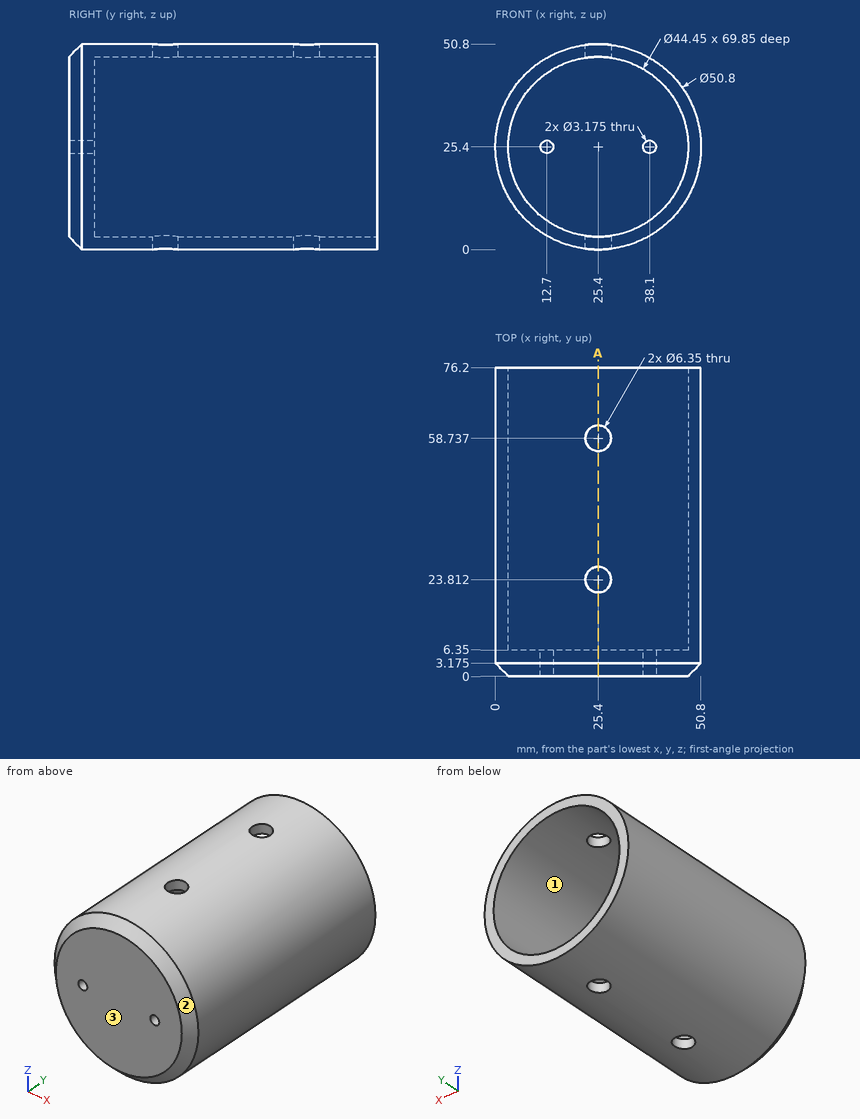
Study the drawing (mm; zero at the part's minimum x, y, z) and answer. Round coordinates to 2 decimals unless told otherwise and drop trailing zeros. Return JSON: item names as keys, results as strings. Group by question number.
Q1. Find the intervals of material crossed by L1, parallel to Y at x = 25.4, z = 2.65 (1 decimal); L2, parallel to Y at x = 12, z = 37; L3, parallel to X at y = 13, z = 5.5 (1 decimal), in increasing order.
Q2. The part is cut by section A-A on x = 25.4. Count the separate pieces of the cut face and the enclosed holes in it.
Q3. The mould has two halves that part along X. Classify the marked faces 1, 2 and 3: released by +X, released by -X, zero draft, split by the parting line, or undercut.
Q4. Each of these flat-tipped pins is pushed along its axis until it touches: pin 1 Ø12 at (x, y) = (36.5, 36.5) entering from +Z; pin 2 Ø22 at (x, z) = (26.5, 24.5) entering from +Y; pin 3 Ø6 at (y, z) = (43, 41.5) entering from -X. Where does it stop, or does it pass through?
Solved:
{
 "1": {"L1": "0.5 to 20.6, 27 to 55.6, 61.9 to 76.2", "L2": "0 to 6.35", "L3": "9.6 to 15.5, 35.3 to 41.2"},
 "2": {"separate pieces": "5", "enclosed holes": "0"},
 "3": {"face 1": "undercut", "face 2": "split by the parting line", "face 3": "zero draft"},
 "4": {"pin 1": "z = 50.28", "pin 2": "y = 6.35", "pin 3": "x = 3.64"}
}
